Work out the finished part from the listing and answer in its coordinate system (mm). A direction names the side the tool comes from. Give positions to 0.01 mm unless a question says otherwise; leave off trailing zeros. Order: outer loops, then holes, each group sorted by start corner. A loop starts at its lowest first (then second) coordinate and runs counter-clockwise, first axis right, second up.
```python
from build123d import *

# Parameters (mm, degrees)
F0_W     = 25
F0_H     = 26.8
F0_R     = 3.5
F1_DEPTH = 3.2
F0_H_2   = 3.2
F2_DEPTH = 30
F4_DEPTH = 3.2
F5_R     = 3.19999
F6_R     = 3.19999


# Not quite as in the source:
# - a fillet or chamfer is up to 0.001 mm smaller than in the source, because OpenCascade refuses the exact size


with BuildPart() as f1:
    # F0 (on Top) → F1 (new body)
    with BuildSketch(Plane.XY):
        with Locations((0, -1.6)):
            Rectangle(F0_W, F0_H)
        with Locations((0, -4.5)):
            Circle(F0_R, mode=Mode.SUBTRACT)
    extrude(amount=F1_DEPTH)

    # F0 (on Top) → F2 (join)
    with BuildSketch(Plane.XY):
        with Locations((0, 13.4)):
            Rectangle(F0_W, F0_H_2)
    extrude(amount=F2_DEPTH)

    # F3 (on face) → F4 (cut)
    with BuildSketch(Plane(origin=(0, 15, 0), x_dir=(-1, 0, 0), z_dir=(0, 1, 0))):
        with BuildLine():
            Line((-3.5, 19.5), (-3.5, 14.5))
            ThreePointArc((-3.5, 14.5), (0, 11), (3.5, 14.5))
            Line((3.5, 14.5), (3.5, 19.5))
            ThreePointArc((3.5, 19.5), (0, 23), (-3.5, 19.5))
        make_face()
    extrude(amount=-F4_DEPTH, mode=Mode.SUBTRACT)

    # F5 (radius 3.2 in the source; OpenCascade refuses exactly that, so slightly less here)
    f5_edges = [f1.edges().sort_by_distance(p)[0] for p in [
        (0, 11.8, 30),
    ]]
    fillet(f5_edges, radius=F5_R)

    # F6 (radius 3.2 in the source; OpenCascade refuses exactly that, so slightly less here)
    f6_edges = [f1.edges().sort_by_distance(p)[0] for p in [
        (0, -15, 3.2),
    ]]
    fillet(f6_edges, radius=F6_R)


solid = f1.part
```
1. The part is cut by section D-D (z = 6.5). Write down the section's boundary in (x, y), then the cut area to 3 significant figures.
Findings below:
outline: (-12.5, 11.8) - (12.5, 11.8) - (12.5, 15) - (-12.5, 15) - close
area: 80.0 mm2
2. Straight lines are drawn through the part: probe 1 along Y at (x, z) = (-10.5, 13.5); probe 2 along Z at (x, y) = (-7.25, -2.5); probe 3 along Z at (x, y) = (3, 12.25). For each, find the intervals that lie inside material, in ascending order.
Findings below:
probe 1: y = 11.8 to 15
probe 2: z = 0 to 3.2
probe 3: z = 0 to 12.7, 21.3 to 28.44
3. Given P1, Ø7, axis at x = -1, y = 1, coming from the +Z side; P2, Ø4, axis at x = 0, y = -4.5, coming from the -Z side; P3, Ø7, axis at x = -1.5, z = 19.5, coming from the -Y side, each flat-ended and moving along its own axis, determine where each tip first touches the part or whether it passes through.
Findings below:
P1: stops at z = 3.2
P2: passes through
P3: stops at y = 11.8
4. The part is cut by section A-A (y = -4.5). Write down the section's boundary in (x, z), then the cut area to 3 significant figures.
Findings below:
outline: (-12.5, 0) - (-3.5, 0) - (-3.5, 3.2) - (-12.5, 3.2) - close; (3.5, 0) - (12.5, 0) - (12.5, 3.2) - (3.5, 3.2) - close
area: 57.6 mm2
5. The mould has two halves that part along X. Classify faces 1 (the face through (-3.5, 13, 17)), 2 (the face through (0.175, 12.713, 29.038)), 3 (the face through (-0.759, -7.917, 1.578)), 4 (the face through (12.5, 7, 3)): pulls with the +X half, pulls with the -X half, needs draft (parallel to the pull), parting line crosses it, or undercut.
Findings below:
face 1: undercut
face 2: needs draft
face 3: undercut
face 4: pulls with the +X half
6. Which of the six approach directions +Z, -Z, +X, -X, +Y, -Y give full straight-line access (tool end or side, diameter ignored) to faces 5 (the face through (0, 0, 3.2)), 6 (the face through (3.5, 13, 17)), 7 (the face through (-3, 15, 11))?
Findings below:
face 5: +Z, +X, -X, -Y
face 6: +Y, -Y
face 7: +Z, -Z, +X, -X, +Y
7. The part is cut by section B-B (x = 0). State how many separate pieces and enclosed holes the cut face has, then the cut area to 3 significant figures.
Findings below:
separate pieces: 3
enclosed holes: 0
area: 117 mm2
